Verification items for the finished model (mm, model axes). Coordinates: 2 decimals unless noted, no trailing zeros. Loops run counter-clockwise (first coordinate to the right, second up) from the corner with the lowest first, then second, coordinate; pieces in that order, holes last. Notation, with made-up numbers: (-18.75, 65.25) - (-10.75, 65.25) arc R22 ccw to (-10.75, 81.25) - close; hole circle Ø1 at (2, 49). An arc over 180 degrees is marked (long way). One line per item, written item: value. Start each with the question number.
(1) Thickness scan on probe 1 along Y at (x, z) = (67.5, 14.25); probe 2 along Y at (x, z) = (78, 18.5). Record the ranges inside material, lowest first. Write a range as [from, to].
(2) Gauge pin test, flat ends, axial feed: P1, Ø5, axis at x = 91.48, y = 0, coming from the -Z side; P2, Ø10, axis at x = 81, z = 3.5, coming from the -Y side. Record the tip position at first contact, or that the pin passes through.
(3) Section check C-C (z = 4.75). Record the boundary of the cut face in (x, y), plus the area to 3 significant figures.
(4) Section check B-B (x = 84). Record the boundary of the cut face in (y, z), plus the area to 3 significant figures.
(5) Draft check along Y on faces 1 (the face through (88, 0, 8)), 2 (the face through (9, 0, 0)), 3 (the face through (3, -15, 10)), 4 (the face through (2, 15, 10)). Enter one of: +Y half, -Y half, draft (parallel to the pull), parting line (faces both ways), or undercut.
(6) Section check A-A (z = 12). Record the boundary of the cut face in (x, y), plus the area to 3 significant figures.
(7) Section check D-D (y = 6). Record the boundary of the cut face in (x, z), plus the area to 3 significant figures.
```python
from build123d import *

# Parameters (mm, degrees)
EXTRUDE_1_DEPTH     = 20
CUT_EXTRUDE_1_DEPTH = 8
SKETCH_4_R          = 1.5
CUT_EXTRUDE_2_DEPTH = 13


with BuildPart() as part:
    # 草图1 → 凸台-拉伸1 (new body)
    with BuildSketch(Plane.XY):
        Polygon((47.5, 15), (103.480762114, 0), (47.5, -15), (-42.5, -15), (-42.5, 15), align=None)
    extrude(amount=EXTRUDE_1_DEPTH)

    # 草图2 → 切除-拉伸1 (cut)
    with BuildSketch(Plane(origin=(0, 0, 0), x_dir=(-1, 0, 0), z_dir=(0, 0, -1))):
        Polygon((-88.480762114, 4.019237886), (-73.480762114, 0), (-88.480762114, -4.019237886), (-103.480762114, 0), align=None)
    extrude(amount=-CUT_EXTRUDE_1_DEPTH, mode=Mode.SUBTRACT)

    # 草图4 → 切除-拉伸2 (cut, through all)
    with BuildSketch(Plane(origin=(0, 0, 8), x_dir=(-1, 0, 0), z_dir=(0, 0, -1))):
        with Locations((-91.480762114, 0)):
            Circle(SKETCH_4_R)
    extrude(amount=-CUT_EXTRUDE_2_DEPTH, mode=Mode.SUBTRACT)


solid = part.part
```
Responses:
1. probe 1: y = [-9.64, 9.64]
1. probe 2: y = [-6.83, 6.83]
2. P1: stops at z = 8
2. P2: stops at y = -7.36
3. outline: (-42.5, -15) - (47.5, -15) - (88.48, -4.02) - (73.48, 0) - (88.48, 4.02) - (47.5, 15) - (-42.5, 15) - close
3. area: 3,420 mm²
4. outline: (-5.22, 0) - (-2.82, 0) - (-2.82, 8) - (2.82, 8) - (2.82, 0) - (5.22, 0) - (5.22, 20) - (-5.22, 20) - close
4. area: 164 mm²
5. face 1: undercut
5. face 2: draft
5. face 3: -Y half
5. face 4: +Y half
6. outline: (-42.5, -15) - (47.5, -15) - (103.48, 0) - (47.5, 15) - (-42.5, 15) - close; hole circle Ø3 at (91.48, 0)
6. area: 3,530 mm²
7. outline: (-42.5, 0) - (81.09, 0) - (81.09, 20) - (-42.5, 20) - close
7. area: 2,470 mm²
